Source: three-view drawing plus pictorial views. Frame: mm from the lowest corner of the part. Give positions to 0.01 mm unless a question says otherwise; leave off trailing zeros. Loops run counter-clockwise (first coordinate to the right, second up) from the corner with the lowest first, then second, coordinate; pieces in that order, holes last. Notation, with made-up numbers: (3.5, 1) - (12.5, 1) arc R14 cw to (12.5, 8) - close; hole circle Ø1 at (59, 28). An arc over 180 degrees is marked (long way). Answer as a JSON object with one key per item and string values. Group by question number.
(1) Section query B-B (x = 55). Return loops of the section in (y, z) (1 decimal).
(2) Section query C-C (x = 20). Return loops of the section in (y, z) (1 decimal), plus the area to 3 significant figures.
(3) Section query A-A (z = 55). Return loops of the section in (x, y), plus the area to 3 significant figures.
(4) Material intervals for L1, parallel to X at y = 1.35, z = 15; L2, parallel to X at y = 3.3, z = 54; L3, parallel to X at y = 3.55, z = 97, sorted ascending.
(5) Section query D-D (z = 91). Return loops of the section in (x, y), plus the area to 3 significant figures.
(6) Pin query (flat end, axial travel): P1, Ø4.5, axis at x = 20, z = 55, coming from the -Y side. Return the tip coordinate at first contact, or that it passes through.
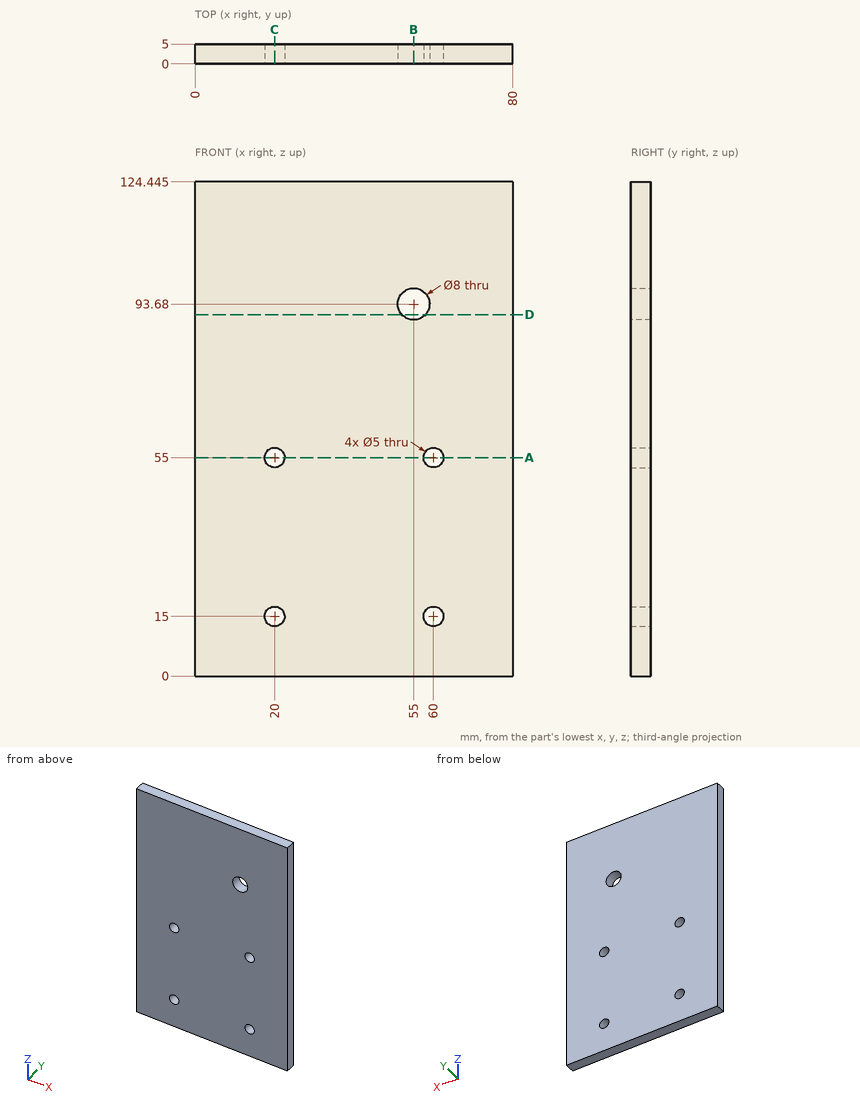
Recorded:
{
 "1": {"outline": "(0, 0) - (5, 0) - (5, 89.7) - (0, 89.7) - close; (0, 97.7) - (5, 97.7) - (5, 124.4) - (0, 124.4) - close"},
 "2": {"outline": "(0, 0) - (5, 0) - (5, 12.5) - (0, 12.5) - close; (0, 17.5) - (5, 17.5) - (5, 52.5) - (0, 52.5) - close; (0, 57.5) - (5, 57.5) - (5, 124.4) - (0, 124.4) - close", "area": "572 mm^2"},
 "3": {"outline": "(0, 0) - (17.5, 0) - (17.5, 5) - (0, 5) - close; (22.5, 0) - (57.5, 0) - (57.5, 5) - (22.5, 5) - close; (62.5, 0) - (80, 0) - (80, 5) - (62.5, 5) - close", "area": "350 mm^2"},
 "4": {"L1": "x = 0 to 17.5, 22.5 to 57.5, 62.5 to 80", "L2": "x = 0 to 17.71, 22.29 to 57.71, 62.29 to 80", "L3": "x = 0 to 52.77, 57.23 to 80"},
 "5": {"outline": "(0, 0) - (52.03, 0) - (52.03, 5) - (0, 5) - close; (57.97, 0) - (80, 0) - (80, 5) - (57.97, 5) - close", "area": "370 mm^2"},
 "6": {"P1": "passes through"}
}
